Verification items for the finished model (mm, model axes). Face numbers are marked on the shaded views. A direction names the side the tool comes from. Round coordinates to 2 decimals unless told otherwise and drop trailing zeros. Write each loop counter-clockwise with the first axis right and the second up, starting at its lowest first coordinate (ties: lowest second). Pieces come first, ordered by that corner, then holes. Notation, with made-up numbers: (6.5, 41) - (33.5, 41) arc R22 ccw to (33.5, 52) - close; hole circle Ø7 at (-36.5, 88.25). An arc over 180 degrees is marked (long way). Write each question's results on one line, items separated by ' | '.
```python
from build123d import *

# Parameters (mm, degrees)
SKETCH1_R           = 10
BOSS_EXTRUDE1_DEPTH = 21
SKETCH2_R           = 1.55
BOSS_EXTRUDE2_DEPTH = 3
SKETCH3_R           = 7.5
BOSS_EXTRUDE3_DEPTH = 6
SKETCH4_R           = 6
CUT_EXTRUDE1_DEPTH  = 25
SKETCH6_R           = 4
CUT_EXTRUDE2_DEPTH  = 1
SKETCH7_R           = 2.5
CUT_EXTRUDE3_DEPTH  = 6
CHAMFER1_SIZE       = 1


with BuildPart() as part:
    # Sketch1 → Boss-Extrude1 (new body)
    with BuildSketch(Plane(origin=(0, 0, 0), x_dir=(1, 0, 0), z_dir=(0, 1, 0))):
        with Locations(Location((0, 0, 0), (0, 0, 90))):
            Circle(SKETCH1_R)
    extrude(amount=BOSS_EXTRUDE1_DEPTH)

    # Sketch2 → Boss-Extrude2 (add)
    with BuildSketch(Plane.XZ):
        with BuildLine():
            Line((-14.361406616, -10), (14.361406616, -10))
            ThreePointArc((14.361406616, -10), (17.5, 0), (14.361406616, 10))
            Line((14.361406616, 10), (-14.361406616, 10))
            ThreePointArc((-14.361406616, 10), (-17.5, 0), (-14.361406616, -10))
        make_face()
        with Locations(Location((-14, 0, 0), (0, 0, 270))):
            Circle(SKETCH2_R, mode=Mode.SUBTRACT)
        with Locations(Location((14, 0, 0), (0, 0, 270))):
            Circle(SKETCH2_R, mode=Mode.SUBTRACT)
    extrude(amount=BOSS_EXTRUDE2_DEPTH)

    # Sketch3 → Boss-Extrude3 (add)
    with BuildSketch(Plane.XZ.offset(3)):
        with Locations(Location((0, 0, 0), (0, 0, 270))):
            Circle(SKETCH3_R)
    extrude(amount=BOSS_EXTRUDE3_DEPTH)

    # Sketch4 → Cut-Extrude1 (cut)
    with BuildSketch(Plane.XZ.offset(9)):
        with Locations(Location((0, 0, 0), (0, 0, 270))):
            Circle(SKETCH4_R)
    extrude(amount=-CUT_EXTRUDE1_DEPTH, mode=Mode.SUBTRACT)

    # Sketch6 → Cut-Extrude2 (cut)
    with BuildSketch(Plane(origin=(10, 0, 0), x_dir=(0, 0, -1), z_dir=(1, 0, 0))):
        with Locations((0, 11.5)):
            Circle(SKETCH6_R)
    extrude(amount=-CUT_EXTRUDE2_DEPTH, mode=Mode.SUBTRACT)

    # Sketch7 → Cut-Extrude3 (cut)
    with BuildSketch(Plane(origin=(9, 0, 0), x_dir=(0, 0, -1), z_dir=(1, 0, 0))):
        with Locations((0, 11.5)):
            Circle(SKETCH7_R)
    extrude(amount=-CUT_EXTRUDE3_DEPTH, mode=Mode.SUBTRACT)

    # Chamfer1
    # the kernel refuses this chamfer: 1 mm, written as the material it adds along each edge
    with BuildSketch(Plane(origin=(0, 0, 0), x_dir=(-2.2377941338409155e-09, 0, 1.0), z_dir=(-1.0, 0, -2.2377941338409155e-09))) as chamfer1_piece_1_section:
        Polygon((10, CHAMFER1_SIZE), (10 + CHAMFER1_SIZE, 0), (10, 0), align=None)
    chamfer1_piece_1 = revolve(axis=Axis((0, 0, 0), (0, 1, 0)), revolution_arc=180.000000128, mode=Mode.PRIVATE)
    chamfer1_piece_1 = split(chamfer1_piece_1, bisect_by=Plane(origin=(10.483044341, 0.483044342, -10), z_dir=(0, 0, 1)), keep=Keep.TOP, mode=Mode.PRIVATE)
    chamfer1_piece_1 = split(chamfer1_piece_1, bisect_by=Plane(origin=(10.483044341, 0.483044342, 10), z_dir=(0, 0, -1)), keep=Keep.TOP, mode=Mode.PRIVATE)
    add(chamfer1_piece_1)
    with BuildSketch(Plane(origin=(0, 0, 0), x_dir=(0, 0, -1), z_dir=(1, 0, 0))) as chamfer1_piece_2_section:
        Polygon((10, CHAMFER1_SIZE), (10 + CHAMFER1_SIZE, 0), (10, 0), align=None)
    chamfer1_piece_2 = revolve(axis=Axis((0, 0, 0), (0, 1, 0)), revolution_arc=179.999999872, mode=Mode.PRIVATE)
    chamfer1_piece_2 = split(chamfer1_piece_2, bisect_by=Plane(origin=(-10.483044341, 0.483044341, -10), z_dir=(0, 0, 1)), keep=Keep.TOP, mode=Mode.PRIVATE)
    chamfer1_piece_2 = split(chamfer1_piece_2, bisect_by=Plane(origin=(-10.483044341, 0.483044341, 10), z_dir=(0, 0, -1)), keep=Keep.TOP, mode=Mode.PRIVATE)
    add(chamfer1_piece_2)
    # the kernel refuses this chamfer: 1 mm, written as the material it takes off along each edge
    with BuildSketch(Plane(origin=(0, 21, 0), x_dir=(0, 0, -1), z_dir=(1, 0, 0))) as chamfer1_2_piece_1:
        Polygon((10, -CHAMFER1_SIZE), (10 - CHAMFER1_SIZE, 0), (10, 0), align=None)
    revolve(axis=Axis((0, 21, 0), (0, 1, 0)), mode=Mode.SUBTRACT)


solid = part.part
```
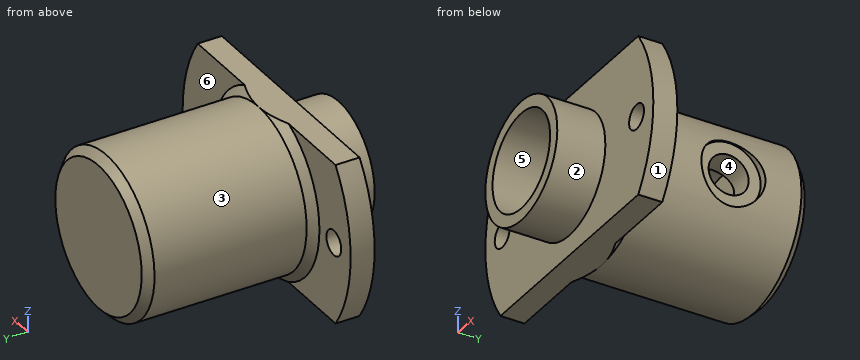
(1) Go/stop test with flat-tipped pins: pin 1 Ø5 at (x, z) = (14, 0) entering from -Y; pin 2 Ø6 at (y, z) = (11.5, 0) entering from -X; pin 3 Ø6 at (x, z) = (0.5, 4.5) entering from -Y; pin 4 Ø6 at (x, y) = (8, 16.5) entering from +Z. Record where each tip stops, or that it passes through.
Answer:
pin 1: y = -3 | pin 2: x = -10 | pin 3: y = -9 | pin 4: z = 8.66
(2) Section check C-C (y = 2.5). Record the cut outline in (x, z), plus the area to 3 significant figures.
Answer:
outline: circle Ø20 at (0, 0); hole circle Ø12 at (0, 0) | area: 201 mm2
(3) Section check A-A (y = -1). Record the cut outline in (x, z), plus the area to 3 significant figures.
Answer:
outline: (-14.36, -10) - (14.36, -10) arc R17.5 ccw to (14.36, 10) - (-14.36, 10) arc R17.5 ccw to start; hole circle Ø3.1 at (-14, 0); hole circle Ø12 at (0, 0); hole circle Ø3.1 at (14, 0) | area: 532 mm2
(4) Mould release check, pull along Z, two halves, no side actions. Record for the marked faces 3, 4, 5 and 6: released by +Z, released by -Z, zero draft, split by the parting line, or undercut.
Answer:
face 3: split by the parting line | face 4: undercut | face 5: undercut | face 6: zero draft
(5) Set-up check for the marked faces 1 and 2: record each of +Z, -Z, +X, -X, +Y, -Y from which the full face is reachable in a straight line by a thin tool's end or side.
Answer:
face 1: +X, +Y, -Y | face 2: -Y
(6) Thickness scan on L1, parallel to Y at x = 6.6, z = 0; L2, parallel to Y at x = -3.5, z = -7; L3, parallel to Y at x = 2, z = -3.5. Record the ranges inside material, lowest first.
Answer:
L1: -9 to 9, 14 to 21 | L2: -3 to 21 | L3: 16 to 21
(7) Section check B-B (x = 13.5). Record the cut outline in (y, z).
Answer:
outline: (-3, -10) - (0, -10) - (0, -1.47) - (-3, -1.47) - close; (-3, 1.47) - (0, 1.47) - (0, 10) - (-3, 10) - close
(8) Section check D-D (y = -6). Record the cut outline in (x, z).
Answer:
outline: circle Ø15 at (0, 0); hole circle Ø12 at (0, 0)
